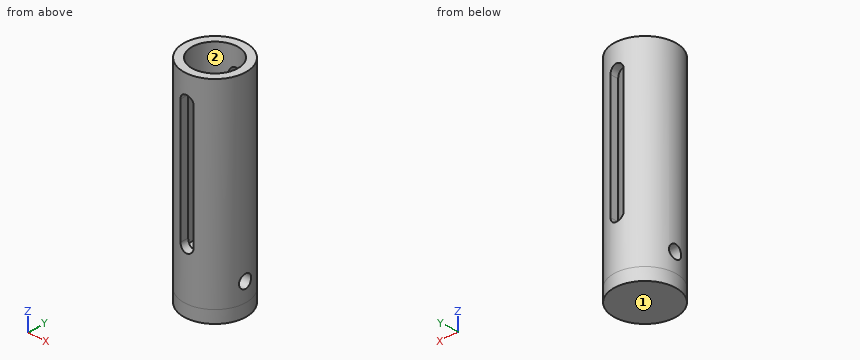
from build123d import *

# Parameters (mm, degrees)
SKETCH1_R                   = 15.875
SKETCH1_R_2                 = 11.7475
BOSS_EXTRUDE1_DEPTH         = 101.6
F_1_4_START                 = 10
F_1_4_CLEARANCE_SLOT1_DEPTH = 7
CUT_EXTRUDE1_REACH          = 106.051
CUT_EXTRUDE1_END_RADIUS     = 15.875
SKETCH7_R                   = 15.875
BOSS_EXTRUDE2_DEPTH         = 15.875
CUT_EXTRUDE3_DEPTH          = 105.050907141
CUT_EXTRUDE3_DEPTH_BACK     = 105.050907141
SKETCH6_R                   = 3.3655
BOSS_EXTRUDE3_START         = 6.35
SKETCH8_R                   = 15.875
BOSS_EXTRUDE3_DEPTH         = 6.35


with BuildPart() as part:
    # Sketch1 → Boss-Extrude1 (new body)
    with BuildSketch(Plane.XY):
        Circle(SKETCH1_R)
        Circle(SKETCH1_R_2, mode=Mode.SUBTRACT)
    extrude(amount=BOSS_EXTRUDE1_DEPTH)

    # 1/4 Clearance Slot1: read off the stored shape, not the designer's step
    # 1/4 Clearance Slot1 outline → 1/4 Clearance Slot1 (cut)
    with BuildSketch(Plane(origin=(0, 0, 0), x_dir=(1, 0, 0), z_dir=(0, 1, 0)).offset(F_1_4_START)):
        with BuildLine():
            Line((3.3782, -88.6968), (3.3782, -25.6032))
            ThreePointArc((3.3782, -25.6032), (0, -22.225), (-3.3782, -25.6032))
            Line((-3.3782, -25.6032), (-3.3782, -88.6968))
            ThreePointArc((-3.3782, -88.6968), (0, -92.075), (3.3782, -88.6968))
        make_face()
    extrude(amount=F_1_4_CLEARANCE_SLOT1_DEPTH, mode=Mode.SUBTRACT)

    # Cut-Extrude1: up to this cylinder (the profile starts inside it)
    cut_extrude1_end = Plane(origin=(0, 0, 57.15), z_dir=(0, 0, -1)) * Cylinder(CUT_EXTRUDE1_END_RADIUS, 244.852, mode=Mode.PRIVATE)
    # Sketch4 → Cut-Extrude1 (cut, up to the surface)
    with BuildSketch(Plane(origin=(0, 0, 0), x_dir=(1, 0, 0), z_dir=(0, 1, 0)), mode=Mode.PRIVATE) as cut_extrude1_sk1:
        with BuildLine():
            Line((-3.3782, -88.6968), (-3.3782, -25.6032))
            ThreePointArc((-3.3782, -25.6032), (0, -22.225), (3.3782, -25.6032))
            Line((3.3782, -25.6032), (3.3782, -88.6968))
            ThreePointArc((3.3782, -88.6968), (0, -92.075), (-3.3782, -88.6968))
        make_face()
    cut_extrude1_tool1 = extrude(cut_extrude1_sk1.sketch, amount=-CUT_EXTRUDE1_REACH, mode=Mode.PRIVATE) & cut_extrude1_end
    add(cut_extrude1_tool1.solids().sort_by_distance((0, 0, 57.15))[0], mode=Mode.SUBTRACT)

    # Sketch7 → Boss-Extrude2 (add)
    with BuildSketch(Plane(origin=(0, 0, 0), x_dir=(-1, 0, 0), z_dir=(0, 0, -1))):
        with Locations(Location((0, 0, 0), (0, 0, 180))):
            Circle(SKETCH7_R)
    extrude(amount=-BOSS_EXTRUDE2_DEPTH)

    # Sketch6 → Cut-Extrude3 (cut, two sides: drawn at the far end of the back side and taken through both)
    with BuildSketch(Plane(origin=(0, 0, 0), x_dir=(0, 0, -1), z_dir=(1, 0, 0)).offset(-CUT_EXTRUDE3_DEPTH_BACK)):
        with Locations((-9.525, 0)):
            Circle(SKETCH6_R)
    extrude(amount=CUT_EXTRUDE3_DEPTH + CUT_EXTRUDE3_DEPTH_BACK, mode=Mode.SUBTRACT)

    # Sketch8 → Boss-Extrude3 (add)
    with BuildSketch(Plane(origin=(0, 0, 0), x_dir=(-1, 0, 0), z_dir=(0, 0, -1)).offset(BOSS_EXTRUDE3_START)):
        Circle(SKETCH8_R)
    extrude(amount=-BOSS_EXTRUDE3_DEPTH)


solid = part.part
Input: part model. Units: mm. Frame: model coordinates. Face numbers are marked on the shaded views. Coordinates: 2 decimals unless noted, no trailing zeros. Answer in a Markdown table with one row per item.
(1) Section query A-A, the plane x = 0. Give the number of separate pieces and of enclosed holes in the cut face, plus the area to 3 significant figures.
Numbers:
| item | result |
|---|---|
| separate pieces | 3 |
| enclosed holes | 1 |
| area | 801 mm^2 |
(2) Draft query along Y for the marked faces 1 and 2. Return one class per face: pulls with the +Y half, pulls with the -Y half, needs draft (parallel to the pull), parting line crosses it, or undercut.
Numbers:
| item | result |
|---|---|
| face 1 | needs draft |
| face 2 | undercut |
(3) Contact query for flat-ended pins moving along their axis: pin 1 Ø3.5 at (y, z) = (-12.5, 45.5) entering from +X; pin 2 Ø8 at (x, z) = (-10.5, 23) entering from +Y; pin 3 Ø1.5 at (x, z) = (-8, 29) entering from +Y. Output: stop coordinate, or through.
Numbers:
| item | result |
|---|---|
| pin 1 | stops at x = 11.68 |
| pin 2 | stops at y = 14.48 |
| pin 3 | stops at y = 14.12 |
(4) Material intervals for line 1 (X direction, y = 0, z = 56.5) (1 decimal); line 2 (Z direction, x = -15, y = -0.5); line 3 (Z direction, x = 4.5, y = 2.5) (3 decimals), sorted ascending. Write a range as [from, to].
Numbers:
| item | result |
|---|---|
| line 1 | x = [-15.9, -11.7], [11.7, 15.9] |
| line 2 | z = [-6.35, 6.2], [12.85, 101.6] |
| line 3 | z = [-6.35, 7.272], [11.778, 15.875] |
